Design review of the part built by this model. Coordinates are the model's own, in mm. Round coordinates to 2 decimals unless told otherwise and drop trailing zeros. Loops run counter-clockwise (first coordinate to the right, second up) from the corner with the lowest first, then second, coordinate; pieces in that order, holes last. Notation, with made-up numbers: (55, 50.25) -> (70, 50.25) arc R22 ccw to (70, 83.25) -> close; hole circle Ø5 at (4, 82.5). An arc over 180 degrees is marked (long way). Answer as CSV lines item,"result". Start each with the question number.
```python
from build123d import *

# Parameters (mm, degrees)
SKETCH1_W            = 101.6
SKETCH1_H            = 76.2
EXTRUDE1_DEPTH       = 1.6002
SKETCH2_R            = 1.778
CUT_EXTRUDE1_DEPTH   = 1.6002
LPATTERN1_COUNT      = 2
LPATTERN1_PITCH      = 63.5
LPATTERN1_COUNT_DIR2 = 2
LPATTERN1_PITCH_DIR2 = 88.9


with BuildPart() as part:
    # Sketch1 → Extrude1 (new body)
    with BuildSketch(Plane.XY):
        with Locations((50.8, -38.1)):
            Rectangle(SKETCH1_W, SKETCH1_H)
    extrude(amount=EXTRUDE1_DEPTH)

    # Sketch2 → Cut-Extrude1 (cut)
    with BuildSketch(Plane.XY.offset(1.6002)):
        with Locations((6.35, -69.85)):
            Circle(SKETCH2_R)
    cut_extrude1 = extrude(amount=-CUT_EXTRUDE1_DEPTH, mode=Mode.SUBTRACT)

    # LPattern1: Cut-Extrude1 2 × 2
    with Locations(*[(j * LPATTERN1_PITCH_DIR2, i * LPATTERN1_PITCH, 0) for i in range(LPATTERN1_COUNT) for j in range(LPATTERN1_COUNT_DIR2) if (i, j) != (0, 0)]):
        add(cut_extrude1, mode=Mode.SUBTRACT)


solid = part.part
```
Q1. For pin 1 Ø6 at (x, y) = (85.5, -20.5) entering from -Z; pin 2 Ø3 at (x, y) = (6.35, -69.85) entering from -Z, all flat-tipped, find the tip position at first contact; note any pin that passes through.
Q2. Add section B-B, the plane y = -69.85. Give the boundary of the cut face in (x, z), and give its area (3 significant figures).
Q3. Mouldability with a two-part tool opening along X and no side actions: class faces 1 (the cylindrical face through (93.474, -6.272, 0.811)), 2 (the flat face through (50, -38, 0)), 3 (the cylindrical face through (93.474, -69.772, 0.811)) as pulls with the +X half, pulls with the -X half, needs draft (parallel to the pull), parting line crosses it, or undercut.
Q4. Add section A-A, the plane x = 95.25. Give the boundary of the cut face in (y, z), and give its area (3 significant figures).
Q5. To check wall thickness, follow probe 1 along X at (y, z) = (-69.85, 1.2); probe 2 along Y at (x, z) = (6.35, 0.95); probe 3 along X at (y, z) = (-69, 0.1). State the ranges of each line that lie inside material, in increasing order. Write a range as from..to.
Worked answers:
1,pin 1,"stops at z = 0"
1,pin 2,"passes through"
2,outline,"(0, 0) -> (4.57, 0) -> (4.57, 1.6) -> (0, 1.6) -> close; (8.13, 0) -> (93.47, 0) -> (93.47, 1.6) -> (8.13, 1.6) -> close; (97.03, 0) -> (101.6, 0) -> (101.6, 1.6) -> (97.03, 1.6) -> close"
2,area,"151 mm^2"
3,face 1,"undercut"
3,face 2,"needs draft"
3,face 3,"undercut"
4,outline,"(-76.2, 0) -> (-71.63, 0) -> (-71.63, 1.6) -> (-76.2, 1.6) -> close; (-68.07, 0) -> (-8.13, 0) -> (-8.13, 1.6) -> (-68.07, 1.6) -> close; (-4.57, 0) -> (0, 0) -> (0, 1.6) -> (-4.57, 1.6) -> close"
4,area,"111 mm^2"
5,probe 1,"x = 0..4.57, 8.13..93.47, 97.03..101.6"
5,probe 2,"y = -76.2..-71.63, -68.07..-8.13, -4.57..0"
5,probe 3,"x = 0..4.79, 7.91..93.69, 96.81..101.6"
